```python
from build123d import *

# Parameters (mm, degrees)
BOSS_EXTRU_1_DEPTH      = 6
ESQUISSE2_R             = 1.25
ENL_V_MAT_EXTRU_1_DEPTH = 10
ESQUISSE4_W             = 20
ESQUISSE4_H             = 6
BOSS_EXTRU_2_DEPTH      = 6


with BuildPart() as part:
    # Esquisse1 → Boss.-Extru.1 (new body)
    with BuildSketch(Plane.XY):
        Polygon((-78, 0), (-78, 124.966679003), (0, 170), (0, 0), align=None)
    extrude(amount=BOSS_EXTRU_1_DEPTH)

    # Esquisse2 → Enlèv. mat.-Extru.1 (cut)
    with BuildSketch(Plane.XY.offset(6)):
        with Locations((-68, 126.121379542)):
            Circle(ESQUISSE2_R)
        with Locations((-50.679491924, 136.121379542)):
            Circle(ESQUISSE2_R)
        with Locations((-16.038475773, 156.121379542)):
            Circle(ESQUISSE2_R)
        with Locations((-33.358983849, 146.121379542)):
            Circle(ESQUISSE2_R)
    extrude(amount=-ENL_V_MAT_EXTRU_1_DEPTH, mode=Mode.SUBTRACT)

    # Esquisse4 → Boss.-Extru.2 (add)
    with BuildSketch(Plane.XZ):
        with Locations((-35, 3)):
            Rectangle(ESQUISSE4_W, ESQUISSE4_H)
    extrude(amount=BOSS_EXTRU_2_DEPTH)


solid = part.part
```
Read the model definition and answer for the solid it produces. Units are mm, in the model's axes. A direction names the side the tool comes from. Round coordinates to 2 decimals unless told otherwise and drop trailing zeros. Write each loop counter-clockwise with the first axis right and the second up, starting at its lowest first coordinate (ties: lowest second). Pieces come first, ordered by that corner, then holes. Notation, with made-up numbers: (-10, 12) - (32, 12) arc R31 ccw to (32, 49) - close; hole circle Ø1 at (74.25, -13.5). An arc over 180 degrees is marked (long way). One line per item, written item: value.
Q1. Straight lines are drawn through the part: line 1 (Y direction, x = -68, z = 3.95); line 2 (Y direction, x = -67, z = 2.75); line 3 (Y direction, x = -14, z = 4.45). For each, find the intervals that lie inside material, in ascending order. Write a range as from..to.
The answers:
line 1: y = 0..124.87, 127.37..130.74
line 2: y = 0..125.37, 126.87..131.32
line 3: y = 0..161.92
Q2. Which of the six approach directions +Z, -Z, +X, -X, +Y, -Y give full straight-line access (tool end or side, diameter ignored) to faces 1 (the flat face through (-39.546, 147.168, 2.958)), 2 (the flat face through (-61, 0, 3)), 3 (the flat face through (-12, 0, 3))?
The answers:
face 1: +Z, -Z, -X, +Y
face 2: +Z, -Z, -X, -Y
face 3: +Z, -Z, +X, -Y
Q3. Find section A-A (z = 1.9). Determine the outline of the cut face in (x, y), and give its area (3 significant figures).
The answers:
outline: (-78, 0) - (-45, 0) - (-45, -6) - (-25, -6) - (-25, 0) - (0, 0) - (0, 170) - (-78, 124.97) - close; hole circle Ø2.5 at (-68, 126.12); hole circle Ø2.5 at (-50.68, 136.12); hole circle Ø2.5 at (-33.36, 146.12); hole circle Ø2.5 at (-16.04, 156.12)
area: 11,600 mm2
Q4. Find section C-C (y = 133). Determine the outline of the cut face in (x, z), and give its area (3 significant figures).
The answers:
outline: (-64.09, 0) - (0, 0) - (0, 6) - (-64.09, 6) - close
area: 385 mm2
Q5. Find section B-B (x = -65). Determine the outline of the cut face in (y, z), and give its area (3 significant figures).
The answers:
outline: (0, 0) - (132.47, 0) - (132.47, 6) - (0, 6) - close
area: 795 mm2
Q6. Each of these flat-tipped pins is pushed along its axis until it touches: P1, Ø3, axis at x = -65.5, z = 1.5, coming from the -Y side; P2, Ø3, axis at y = -2, z = 3.5, coming from the +X side; P3, Ø2, axis at x = -50.68, y = 136.12, coming from the +Z side. Where does it stop, or does it pass through?
The answers:
P1: stops at y = 0
P2: stops at x = -25
P3: passes through
